from build123d import *

# Parameters (mm, degrees)
SKETCH_R        = 22.5
PAD_DEPTH       = 8
SKETCH001_R     = 8.75
PAD001_DEPTH    = 20.5
SKETCH002_R     = 6
SKETCH002_R_2   = 5
PAD002_DEPTH    = 13
FILLET_R        = 6.99
FILLET001_R     = 4.5
POCKET_DEPTH    = 4.5
FILLET002_R     = 1.5
SKETCH008_R     = 2.5
POCKET001_DEPTH = 18
SKETCH009_W     = 10
SKETCH009_H     = 10
SKETCH009_R     = 0.005
PAD007_DEPTH    = 0.1


with BuildPart() as part:
    # Sketch (on XY_Plane of Origin) → Pad (new body)
    with BuildSketch(Plane.XY):
        Circle(SKETCH_R)
    extrude(amount=PAD_DEPTH)

    # Sketch001 (on XY_Plane of Origin) → Pad001 (join)
    with BuildSketch(Plane.XY):
        Circle(SKETCH001_R)
    extrude(amount=PAD001_DEPTH)

    # Sketch002 (on XY_Plane of Origin) → Pad002 (join)
    with BuildSketch(Plane.XY):
        Circle(SKETCH002_R)
        Circle(SKETCH002_R_2, mode=Mode.SUBTRACT)
    extrude(amount=PAD002_DEPTH)

    # Fillet
    fillet_edges = [part.edges().sort_by_distance(p)[0] for p in [
        (-8.75, 0, 8),
    ]]
    fillet(fillet_edges, radius=FILLET_R)

    # Fillet001
    fillet001_edges = [part.edges().sort_by_distance(p)[0] for p in [
        (-22.5, 0, 0),
    ]]
    fillet(fillet001_edges, radius=FILLET001_R)

    # Sketch003 (on XY_Plane of Origin) → Pocket (cut)
    with BuildSketch(Plane.XY.offset(6)):
        Polygon((4.25, 2.453739), (0, 4.907477), (-4.25, 2.453739), (-4.25, -2.453739), (0, -4.907477), (4.25, -2.453739), align=None)
    extrude(amount=POCKET_DEPTH, mode=Mode.SUBTRACT)

    # Fillet002
    fillet002_edges = [part.edges().sort_by_distance(p)[0] for p in [
        (-22.5, 0, 8),
    ]]
    fillet(fillet002_edges, radius=FILLET002_R)

    # Sketch008 (on XY_Plane of Origin) → Pocket001 (cut)
    with BuildSketch(Plane.XY.offset(3)):
        Circle(SKETCH008_R)
    extrude(amount=POCKET001_DEPTH, mode=Mode.SUBTRACT)

    # Sketch009 (on XY_Plane of Origin) → Pad007 (join)
    with BuildSketch(Plane.XY.offset(10.5)):
        Rectangle(SKETCH009_W, SKETCH009_H)
        Circle(SKETCH009_R, mode=Mode.SUBTRACT)
    extrude(amount=PAD007_DEPTH)


solid = part.part
The model under review builds one solid part; all positions refer to its coordinate system, in mm. A direction names the side the tool comes from. Coordinates: 2 decimals unless noted, no trailing zeros. Use a Markdown table: item, result. Add a question column.
1. Draft analysis for pull direction Y (two halves, no side actions). For faces 4 (the face through (10.382, -19.961, 5.486)), 5 (the face through (0, 0, 0)), 6 (the face through (4.25, 0, 8)), state which applies: pulls with the +Y half, pulls with the -Y half, needs draft (parallel to the pull), parting line crosses it, or undercut.
2. To check wall thickness, follow line 1 (Y direction, x = 0, z = 17.75); line 2 (Y direction, x = 0, z = 4.25); line 3 (Z direction, x = 11, y = 11.5). State the ranges of each line that lie inside material, in increasing order.
3. Machinability: for faces 1 (the face through (2.095, -3.698, 8.218)), 2 (the face through (-2, 16, 8)), 3 (the face through (2, -2, 20.5)), which of the approach directions +Z, -Z, +X, -X, +Y, -Y give a long, thin tool a straight path to every point of the face, cutting with its end or side? Answer none if there is none.
4. Clearance check with flat-ended pins moving along their axes: pin 1 Ø5 at (x, z) = (-15, 5.5) entering from +Y; pin 2 Ø1.3 at (y, z) = (0, 8) entering from -X; pin 3 Ø1.3 at (y, z) = (-0.5, 8) entering from +X; pin 4 Ø1.5 at (x, y) = (-0.5, -1) entering from -Z. State where each tip first meets the part, or that it passes through.
Returned:
| question | item | result |
|---|---|---|
| 1 | face 4 | parting line crosses it |
| 1 | face 5 | needs draft |
| 1 | face 6 | undercut |
| 2 | line 1 | y = -8.75 to -2.5, 2.5 to 8.75 |
| 2 | line 2 | y = -22.49 to -2.5, 2.5 to 22.49 |
| 2 | line 3 | z = 0 to 8 |
| 3 | face 1 | none |
| 3 | face 2 | +Z |
| 3 | face 3 | +Z, +X, -X, +Y, -Y |
| 4 | pin 1 | stops at y = 18.71 |
| 4 | pin 2 | stops at x = -22.24 |
| 4 | pin 3 | stops at x = 22.23 |
| 4 | pin 4 | stops at z = 0 |
